Build history of the part. All positions in model axes, mm. A direction names the side the tool comes from. Round coordinates to 2 decimals unless told otherwise and drop trailing zeros. Write each loop counter-clockwise with the first axis right and the second up, starting at its lowest first coordinate (ties: lowest second). Pieces come first, ordered by that corner, then holes. Notation, with made-up numbers: (81.25, -8) -> (89.25, -8) arc R32 cw to (89.25, 31) -> close; hole circle Ø4 at (-14.75, 59.25). An arc over 180 degrees is marked (long way). One line per question, with ' | ' between items.
Autodesk Inventor part; units mm, degrees
ref_plane "YZ Plane" through (0, 0, 0) normal (1, 0, 0) x (0, 1, 0)
ref_plane "XZ Plane" through (0, 0, 0) normal (0, 1, 0) x (-1, 0, 0)
ref_plane "XY Plane" through (0, 0, 0) normal (0, 0, 1) x (1, 0, 0)
sketch "スケッチ1" plane through (0, 0, 0) normal (1, 0, 0) x (0, 1, 0)
  line L0 (21.98, 0) -> (21.98, 2.5)
  line L1 (21.98, 2.5) -> (19.98, 2.5)
  line L2 (19.98, 2.5) -> (19.98, 9.5)
  line L3 (19.98, 9.5) -> (0, 9.5)
  line L4 (0, 9.5) -> (0, 0)
  line L5 (0, 0) -> (21.98, 0)
  dimension "d0" = 19.98
  dimension "d1" = 7
  dimension "d2" = 2.5
  dimension "d3" = 2
revolve "回転1" add sketch "スケッチ1" angle 360 about axis through (0, 0, 9.5) along (0, 0, -1)
chamfer "面取り1" distance 0.5 angle 45 1 edges at (0, -19.98, 9.5)
sketch "スケッチ4" plane through (0, 0, 9.5) normal (0, 0, 1) x (1, 0, 0)
  circle A0 centre (0, 0) radius 12.5
  point P0 (0, 0)
  point P1 (0, 12.5)
  point P2 (-12.5, 0)
  point P3 (0, -12.5)
  point P4 (12.5, 0)
  dimension "d13" = 25
  dimension "d16" = 360
hole "穴1" at (0, 12.5, 9.5) at (-12.5, 0, 9.5) at (0, -12.5, 9.5) at (12.5, 0, 9.5) direction (0, 0, -1) diameter 3.2 end through all
sketch "スケッチ5" plane through (0, 0, 9.5) normal (0, 0, 1) x (1, 0, 0)
  circle A0 centre (0, 0) radius 16.15
  point P0 (0, 0)
  dimension "d30" = 32.3
extrude "押し出し4" cut sketch "スケッチ5" against normal blind 5.5
chamfer "面取り2" distance 0.5 angle 45 1 edges at (-16.15, 0, 9.5)
properties part number "base13" material "ABS プラスチック"
(1) 3-axis set-ups, long thin cutter, end or side, ignore diameter. For faces 1 (the flat face through (0, 0, 4)), 2 (the cylindrical face through (-14.086, 0.208, 1.972)): which of +Z, -Z, +X, -X, +Y, -Y reach the whole face in a straight line?
Calculated:
face 1: +Z | face 2: +Z, -Z
(2) Wall check: line 1 (X direction, y = 0, z = 2.35); line 2 (Z direction, x = -9, y = -11); line 3 (Y direction, x = 6.5, z = 8). Give the ranges that are in metal, low to high. Write a range as from..to.
Calculated:
line 1: -21.98..-14.1, -10.9..10.9, 14.1..21.98 | line 2: 0..4 | line 3: -18.89..-14.78, 14.78..18.89
(3) Slice it at B-B (z = 5). Write the cut outline in (x, y).
Calculated:
outline: circle Ø39.96 at (0, 0); hole circle Ø32.3 at (0, 0)
(4) Slice it at A-A (y = 0). Write the cut outline in (x, z).
Calculated:
outline: (-21.98, 0) -> (-14.1, 0) -> (-14.1, 4) -> (-16.15, 4) -> (-16.15, 9) -> (-16.65, 9.5) -> (-19.48, 9.5) -> (-19.98, 9) -> (-19.98, 2.5) -> (-21.98, 2.5) -> close; (-10.9, 0) -> (10.9, 0) -> (10.9, 4) -> (-10.9, 4) -> close; (14.1, 0) -> (21.98, 0) -> (21.98, 2.5) -> (19.98, 2.5) -> (19.98, 9) -> (19.48, 9.5) -> (16.65, 9.5) -> (16.15, 9) -> (16.15, 4) -> (14.1, 4) -> close
(5) Mould opens along X. For faces 3 (the cylindrical face through (19.505, -4.331, 5.796)), 4 (the flat face through (-18, 10, 2.5)), 5 (the cylindrical face through (-3.501, -15.766, 6.535)) say: pulls with the +X half, pulls with the -X half, needs draft (parallel to the pull), parting line crosses it, or undercut.
Calculated:
face 3: parting line crosses it | face 4: needs draft | face 5: undercut
(6) Drop flat-ended pins along their axis: pin 1 (1 mm diameter, centred on x = 8, z = 4, fed in from +Y); pin 2 (2.5 mm diameter, centred on x = -12.5, y = 0, fed in from -Z); pin 3 (5 mm diameter, centred on x = 11.5, z = 6, fed in from +Y); pin 4 (5 mm diameter, centred on x = -16.5, z = 8, fed in from -Y). Give the stop position or say it passes through.
Calculated:
pin 1: y = 18.52 | pin 2: through | pin 3: y = 17.84 | pin 4: y = -14.25
